For this review, take the finished solid that the model builds, in its own axes (mm). A direction names the side the tool comes from. Coordinates: 2 decimals unless noted, no trailing zeros. Order: outer loops, then holes, each group sorted by start corner. A loop starts at its lowest first (then second) coordinate and runs counter-clockwise, first axis right, second up. Notation, with made-up numbers: (82.25, 55.5) -> (90.25, 55.5) arc R29 cw to (90.25, 90.5) -> close; hole circle Ø8 at (46.5, 1.5). An arc over 180 degrees is marked (long way). Return JSON: item names as keys, results as strings. Group by question number.
Item 1: Machinability: for faces 4 (the flat face through (15, 63.5, 6)), 5 (the flat face through (0, 5, -9.525)), 6 (the flat face through (11.349, 71, -19)), which of the approach directions +Z, -Z, +X, -X, +Y, -Y give a long, thin tool a straight path to every point of the face, cutting with its end or side? Answer none if there is none.
Item 2: Take a section at C-C (z = -5). Write out the cut boundary in (x, y) (3 decimals).
Item 3: Take a section at B-B (x = -10.5). Write out the cut boundary in (y, z) (3 decimals).
Item 4: For line 1 along Y through (x, z) = (9.5, -1); line 2 along Z through (x, y) = (0, 3) (3 decimals); line 3 along Z through (x, y) = (-11.5, 13.5), list the stretches that pass through material, from the lowest coordinate up.
Item 5: Draft analysis for pull direction Z (two halves, no side actions). For faces 1 (the flat face through (15, 71, -25.4)), 2 (the flat face through (0, 9.525, -6)), 3 (the flat face through (11.349, 71, 6)), state which applies: +Z half, -Z half, draft (parallel to the pull), parting line (faces both ways), or undercut.
Item 6: Take a section at D-D (y = 66.5). Write out the cut boundary in (x, z), then the cut area to 3 significant figures.
Item 7: Insertion check: pin 1 (12 mm diameter, centred on x = 7.5, y = 49.5, fed in from -Z); pin 2 (2.5 mm diameter, centred on x = -9.52, y = 4.76, fed in from -Z); pin 3 (10 mm diameter, centred on y = 23.5, z = 2.5, fed in from +X); pin 4 (4 mm diameter, centred on y = 75, z = 4, fed in from -X). Each pin has a flat end and moves straight along its axis. Give the tip position at first contact, or say it passes through.
Item 8: Take a section at A-A (y = 8.5). Write out the cut boundary in (x, z) (3 decimals), then the cut area to 3 significant figures.
```python
from build123d import *

# Parameters (mm, degrees)
BOSS_EXTRUDE1_DEPTH   = 12.7
SKETCH5_W             = 6.35
SKETCH5_H             = 9.525
CUT_EXTRUDE1_DEPTH    = 35.925
F_6_CLEARANCE_HOLE1_D = 3.7973
SKETCH9_W             = 7.701365702
SKETCH9_H             = 15.24
BOSS_EXTRUDE2_DEPTH   = 19.05


with BuildPart() as part:
    # Sketch1 → Boss-Extrude1 (new body)
    with BuildSketch(Plane.XY):
        with BuildLine():
            Line((-15.875, 0), (15.875, 0))
            Line((15.875, 0), (15.875, 9.525))
            ThreePointArc((15.875, 9.525), (6.228979432, 37.173295328), (19.05, 63.5))
            Line((19.05, 63.5), (19.05, 78.74))
            Line((19.05, 78.74), (11.348634298, 78.74))
            ThreePointArc((11.348634298, 78.74), (-8.824454666, 46.71317853), (-15.875, 9.525))
            Line((-15.875, 9.525), (-15.875, 0))
        make_face()
    extrude(amount=-BOSS_EXTRUDE1_DEPTH)

    # Sketch5 → Cut-Extrude1 (cut, through all)
    with BuildSketch(Plane.ZY.offset(15.875)):
        with Locations((-6.35, 4.7625)):
            Rectangle(SKETCH5_W, SKETCH5_H)
    extrude(amount=-CUT_EXTRUDE1_DEPTH, mode=Mode.SUBTRACT)

    # #6 Clearance Hole1 (through all)
    with Locations(Plane.XY):
        with Locations((9.525, 4.7625), (-9.525, 4.7625)):
            Hole(F_6_CLEARANCE_HOLE1_D / 2)

    # Sketch9 → Boss-Extrude2 (add, symmetric)
    with BuildSketch(Plane.XY.offset(-6.35)):
        with Locations((15.199317149, 71.12)):
            Rectangle(SKETCH9_W, SKETCH9_H)
    extrude(amount=BOSS_EXTRUDE2_DEPTH, both=True)


solid = part.part
```
Findings below:
{
 "1": {"face 4": "+Z, +X, -X, -Y", "face 5": "+X, -X, -Y", "face 6": "-Z, -X, +Y, -Y"},
 "2": {"outline": "(-15.875, 9.525) -> (15.875, 9.525) arc R38.1 cw to (19.05, 63.5) -> (19.05, 78.74) -> (11.349, 78.74) arc R101.6 ccw to start"},
 "3": {"outline": "(0, -12.7) -> (3.133, -12.7) -> (3.133, -9.525) -> (0, -9.525) -> close; (0, -3.175) -> (3.133, -3.175) -> (3.133, 0) -> (0, 0) -> close; (6.392, -12.7) -> (42.133, -12.7) -> (42.133, 0) -> (6.392, 0) -> (6.392, -3.175) -> (9.525, -3.175) -> (9.525, -9.525) -> (6.392, -9.525) -> close"},
 "4": {"line 1": "y = 0 to 2.86, 6.66 to 19.34, 50.53 to 76.7", "line 2": "z = -12.7 to -9.525, -3.175 to 0", "line 3": "z = -12.7 to 0"},
 "5": {"face 1": "-Z half", "face 2": "undercut", "face 3": "draft"},
 "6": {"outline": "(1.6, -12.7) -> (11.35, -12.7) -> (11.35, -25.4) -> (19.05, -25.4) -> (19.05, 12.7) -> (11.35, 12.7) -> (11.35, 0) -> (1.6, 0) -> close", "area": "417 mm2"},
 "7": {"pin 1": "stops at z = -12.7", "pin 2": "passes through", "pin 3": "stops at x = 9.58", "pin 4": "stops at x = 11.35"},
 "8": {"outline": "(-15.875, -12.7) -> (15.875, -12.7) -> (15.875, -9.525) -> (-15.875, -9.525) -> close; (-15.875, -3.175) -> (15.875, -3.175) -> (15.875, 0) -> (-15.875, 0) -> close", "area": "202 mm2"}
}
